from build123d import *

# Parameters (mm, degrees)
BOSS_EXTRU_1_DEPTH = 7
ESQUISSE1_4_R      = 19
BOSS_EXTRU_2_DEPTH = 3


with BuildPart() as part:
    # Esquisse1 → Boss.-Extru.1 (new body)
    with BuildSketch(Plane.XY):
        with BuildLine():
            ThreePointArc((-9.5, 7.331439149), (-6.607434253, 10.01707605), (-3, 11.618950039))
            Line((-3, 11.618950039), (-3, 14.696938457))
            ThreePointArc((-3, 14.696938457), (-11.618950039, 9.486832981), (-15, 0))
            Line((-15, 0), (-12, 0))
            ThreePointArc((-12, 0), (-11.357816692, 3.872983346), (-9.5, 7.331439149))
        make_face()
        with BuildLine():
            Line((-12, 0), (-15, 0))
            ThreePointArc((-15, 0), (-11.291589791, -9.874208829), (-2, -14.866068747))
            Line((-2, -14.866068747), (-2, -11.832159566))
            ThreePointArc((-2, -11.832159566), (-6.174675786, -10.289479041), (-9.5, -7.331439149))
            ThreePointArc((-9.5, -7.331439149), (-11.357816692, -3.872983346), (-12, 0))
        make_face()
        with BuildLine():
            ThreePointArc((2, -14.866068747), (11.291589791, -9.874208829), (15, 0))
            Line((15, 0), (12, 0))
            ThreePointArc((12, 0), (11.357816692, -3.872983346), (9.5, -7.331439149))
            ThreePointArc((9.5, -7.331439149), (6.174675786, -10.289479041), (2, -11.832159566))
            Line((2, -11.832159566), (2, -14.866068747))
        make_face()
        with BuildLine():
            ThreePointArc((-2, -14.866068747), (0, -15), (2, -14.866068747))
            Line((2, -14.866068747), (2, -11.832159566))
            ThreePointArc((2, -11.832159566), (0, -12), (-2, -11.832159566))
            Line((-2, -11.832159566), (-2, -14.866068747))
        make_face()
        with BuildLine():
            Line((3, 14.696938457), (3, 11.618950039))
            ThreePointArc((3, 11.618950039), (6.607434253, 10.01707605), (9.5, 7.331439149))
            ThreePointArc((9.5, 7.331439149), (11.357816692, 3.872983346), (12, 0))
            Line((12, 0), (15, 0))
            ThreePointArc((15, 0), (11.618950039, 9.486832981), (3, 14.696938457))
        make_face()
        with BuildLine():
            ThreePointArc((-3, 11.618950039), (0, 12), (3, 11.618950039))
            Line((3, 11.618950039), (3, 14.696938457))
            ThreePointArc((3, 14.696938457), (0, 15), (-3, 14.696938457))
            Line((-3, 14.696938457), (-3, 11.618950039))
        make_face()
        with BuildLine():
            Line((-9.5, 0), (-9.5, 7.331439149))
            ThreePointArc((-9.5, 7.331439149), (-11.357816692, 3.872983346), (-12, 0))
            Line((-12, 0), (-9.5, 0))
        make_face()
        with BuildLine():
            Line((-9.5, -7.331439149), (-9.5, 0))
            Line((-9.5, 0), (-12, 0))
            ThreePointArc((-12, 0), (-11.357816692, -3.872983346), (-9.5, -7.331439149))
        make_face()
        with BuildLine():
            ThreePointArc((12, 0), (11.357816692, 3.872983346), (9.5, 7.331439149))
            Line((9.5, 7.331439149), (9.5, 0))
            Line((9.5, 0), (12, 0))
        make_face()
        with BuildLine():
            Line((12, 0), (9.5, 0))
            Line((9.5, 0), (9.5, -7.331439149))
            ThreePointArc((9.5, -7.331439149), (11.357816692, -3.872983346), (12, 0))
        make_face()
    extrude(amount=BOSS_EXTRU_1_DEPTH)

    # Esquisse1_4 → Boss.-Extru.2 (add)
    with BuildSketch(Plane.XY):
        Circle(ESQUISSE1_4_R)
        with BuildLine():
            ThreePointArc((-9.5, 7.331439149), (0, 12), (9.5, 7.331439149))
            Line((9.5, 7.331439149), (9.5, -7.331439149))
            ThreePointArc((9.5, -7.331439149), (0, -12), (-9.5, -7.331439149))
            Line((-9.5, -7.331439149), (-9.5, 7.331439149))
        make_face(mode=Mode.SUBTRACT)
    extrude(amount=-BOSS_EXTRU_2_DEPTH)


solid = part.part
Source: CAD feature listing. Evaluate the final solid. Frame: model axes, mm. A direction names the side the tool comes from. Round coordinates to 2 decimals unless told otherwise and drop trailing zeros. Write each loop counter-clockwise with the first axis right and the second up, starting at its lowest first coordinate (ties: lowest second). Pieces come first, ordered by that corner, then holes. Notation, with made-up numbers: (20, 75.25) - (60, 75.25) arc R12 cw to (60, 91.25) - close; hole circle Ø3 at (69, 48). An arc over 180 degrees is marked (long way). Use CSV: the item, a comma, the result in double quotes. Start each with the question number.
(1) Mould query, pull axis X, two halves, no side actions, for faces 4 (the face through (8.767, -16.856, -1.479)), 5 (the face through (10, 0, 7)), 6 (the face through (9.5, 0, 2)). Classes: pulls with the +X half, pulls with the -X half, needs draft (parallel to the pull), parting line crosses it, or undercut.
(2) Cut plane A-A, the plane x = 0. Return loops of the section in (y, z).
(3) Material intervals for probe 1 along X at (y, z) = (-0.5, -1); probe 2 along X at (y, z) = (0, 1.75); probe 3 along Y at (x, z) = (-3.5, 3.5), sorted ascending. Write a range as [from, to].
(4) First-contact query: pin 1 Ø3 at (y, z) = (11, 3) entering from +X; pin 2 Ø6 at (y, z) = (-8, -0.5) entering from -X; pin 3 Ø5 at (y, z) = (-3, 4.5) entering from -X. Flat tips, straight axial feed; report the tip coordinate or a pass-through.
(5) Set-up query: faces 1 (the face through (-0.3, -12.4, -3)), 2 (the face through (-9.5, 0, 2)), 3 (the face through (14, 6, 0)). Return all of +Z, -Z, +X, -X, +Y, -Y with unobstructed straight access to the full face (end or side cutting, diameter ignored); none if empty.
(6) Cut plane B-B, the plane z = -2.25. Return loops of the section in (x, y), and give its area (3 significant figures).
(7) Cut plane C-C, the plane y = 0.5. Return loops of the section in (x, z).
(8) Cut plane D-D, the plane x = -5. Return loops of the section in (y, z), and give its area (3 significant figures).
Geometry says:
1,face 4,"parting line crosses it"
1,face 5,"needs draft"
1,face 6,"undercut"
2,outline,"(-19, -3) - (-12, -3) - (-12, 7) - (-15, 7) - (-15, 0) - (-19, 0) - close; (12, -3) - (19, -3) - (19, 0) - (15, 0) - (15, 7) - (12, 7) - close"
3,probe 1,"[-18.99, -9.5], [9.5, 18.99]"
3,probe 2,"[-15, -9.5], [9.5, 15]"
3,probe 3,"[-14.59, -11.48], [11.48, 14.59]"
4,pin 1,"x = 11.61"
4,pin 2,"x = -18.33"
4,pin 3,"x = -14.99"
5,face 1,"-Z, +X, -X, +Y, -Y"
5,face 2,"+Z, -Z"
5,face 3,"+Z"
6,outline,"circle Ø38 at (0, 0); hole (-9.5, -7.33) arc R12 ccw to (9.5, -7.33) - (9.5, 7.33) arc R12 ccw to (-9.5, 7.33) - close"
6,area,"732 mm²"
7,outline,"(-18.99, -3) - (-9.5, -3) - (-9.5, 7) - (-14.99, 7) - (-14.99, 0) - (-18.99, 0) - close; (9.5, -3) - (18.99, -3) - (18.99, 0) - (14.99, 0) - (14.99, 7) - (9.5, 7) - close"
8,outline,"(-18.33, -3) - (-10.91, -3) - (-10.91, 7) - (-14.14, 7) - (-14.14, 0) - (-18.33, 0) - close; (10.91, -3) - (18.33, -3) - (18.33, 0) - (14.14, 0) - (14.14, 7) - (10.91, 7) - close"
8,area,"89.8 mm²"
